```python
from build123d import *

# Parameters (mm, degrees)
BOSS_EXTRUDE1_DEPTH = 1.4
SKETCH2_R           = 1.5
BOSS_EXTRUDE2_DEPTH = 10
SKETCH3_R           = 1.9
BOSS_EXTRUDE3_DEPTH = 1
FILLET1_R           = 0.4


with BuildPart() as part:
    # Sketch1 → Boss-Extrude1 (new body)
    with BuildSketch(Plane(origin=(0, 0, 0), x_dir=(1, 0, 0), z_dir=(0, 1, 0))):
        with BuildLine():
            Line((-1.5, 2), (1.5, 2))
            ThreePointArc((1.5, 2), (3.5, 0), (1.5, -2))
            Line((1.5, -2), (-1.5, -2))
            ThreePointArc((-1.5, -2), (-3.5, 0), (-1.5, 2))
        make_face()
    extrude(amount=BOSS_EXTRUDE1_DEPTH)

    # Sketch2 → Boss-Extrude2 (add)
    with BuildSketch(Plane(origin=(0, 0, 0), x_dir=(-1, 0, 0), z_dir=(0, -1, 0))):
        with Locations(Location((0, 0, 0), (0, 0, 90))):
            Circle(SKETCH2_R)
    extrude(amount=BOSS_EXTRUDE2_DEPTH)

    # Sketch3 → Boss-Extrude3 (add)
    with BuildSketch(Plane(origin=(0, -9.2, 0), x_dir=(-1, 0, 0), z_dir=(0, -1, 0))):
        with Locations(Location((0, 0, 0), (0, 0, 90))):
            Circle(SKETCH3_R)
    extrude(amount=-BOSS_EXTRUDE3_DEPTH)

    # Fillet1
    fillet1_edges = [part.edges().sort_by_distance(p)[0] for p in [
        (3.5, 1.4, 0),
        (0, 1.4, -2),
        (-3.5, 1.4, 0),
        (0, 1.4, 2),
    ]]
    fillet(fillet1_edges, radius=FILLET1_R)


solid = part.part
```
The listing builds one solid part. Answer for the finished solid, in the listing's coordinates (mm). A direction names the side the tool comes from. Round coordinates to 2 decimals unless told otherwise and drop trailing zeros. Write each loop counter-clockwise with the first axis right and the second up, starting at its lowest first coordinate (ties: lowest second). Pieces come first, ordered by that corner, then holes. Notation, with made-up numbers: (64.5, 3) -> (102.5, 3) arc R27 ccw to (102.5, 35) -> close; hole circle Ø5 at (52.25, 78). An arc over 180 degrees is marked (long way). Use CSV: the item, a comma, the result in double quotes. Start each with the question number.
(1) The mould has two halves that part along Y. Classify faces 3 (the face through (0, 1.4, 0)), 4 (the face through (-0.728, -8.707, -1.755)), 5 (the face through (-2, 0, 0)), 6 (the face through (0.45, -4.04, -1.43)): released by +Y, released by -Y, zero draft, split by the parting line, or undercut.
(2) Which of the six approach directions +Z, -Z, +X, -X, +Y, -Y give full straight-line access (tool end or side, diameter ignored) to faces 1 (the face through (0.45, -9.59, -1.43)), 2 (the face through (3.5, 0.5, 0))?
(3) Each of these flat-tipped pins is pushed along its axis until it touches: pin 1 (2 mm diameter, centred on x = 1, y = -4, fed in from +Z); pin 2 (2 mm diameter, centred on y = -7.5, z = -1.5, fed in from +X). Where does it stop, or does it pass through?
(4) Section C-C on y = -0.5 is taken. Give the vertices of the cut face in (x, z).
(5) Section B-B on x = 0 is taken. Give the vertices of the cut face in (y, z), then the cut area to 3 significant figures.
(6) Consider L1, parallel to Y at x = -1, z = 1.4; L2, parallel to Y at x = 2.25, z = -1.35; L3, parallel to X at y = -1.5, z = 0.1. Determine where each line is inside the solid, lowest interval first. Write a range as from..to.
(7) Section A-A on z = 0 is taken. Give the vertices of the cut face in (x, y), then the cut area to 3 significant figures.
A:
1,face 3,"released by +Y"
1,face 4,"zero draft"
1,face 5,"undercut"
1,face 6,"undercut"
2,face 1,"-Y"
2,face 2,"+X, +Y, -Y"
3,pin 1,"stops at z = 1.5"
3,pin 2,"stops at x = 1.73"
4,outline,"circle Ø3 at (0, 0)"
5,outline,"(-10, -1.5) -> (-9.2, -1.5) -> (-9.2, -1.9) -> (-8.2, -1.9) -> (-8.2, -1.5) -> (0, -1.5) -> (0, -2) -> (1, -2) arc R0.4 ccw to (1.4, -1.6) -> (1.4, 1.6) arc R0.4 ccw to (1, 2) -> (0, 2) -> (0, 1.5) -> (-8.2, 1.5) -> (-8.2, 1.9) -> (-9.2, 1.9) -> (-9.2, 1.5) -> (-10, 1.5) -> close"
5,area,"36.3 mm²"
6,L1,"y = -9.2..-8.2, 0..1.4"
6,L2,"y = 0..1.4"
6,L3,"x = -1.5..1.5"
7,outline,"(-3.5, 0) -> (-1.5, 0) -> (-1.5, -8.2) -> (-1.9, -8.2) -> (-1.9, -9.2) -> (-1.5, -9.2) -> (-1.5, -10) -> (1.5, -10) -> (1.5, -9.2) -> (1.9, -9.2) -> (1.9, -8.2) -> (1.5, -8.2) -> (1.5, 0) -> (3.5, 0) -> (3.5, 1) arc R0.4 ccw to (3.1, 1.4) -> (-3.1, 1.4) arc R0.4 ccw to (-3.5, 1) -> close"
7,area,"40.5 mm²"
